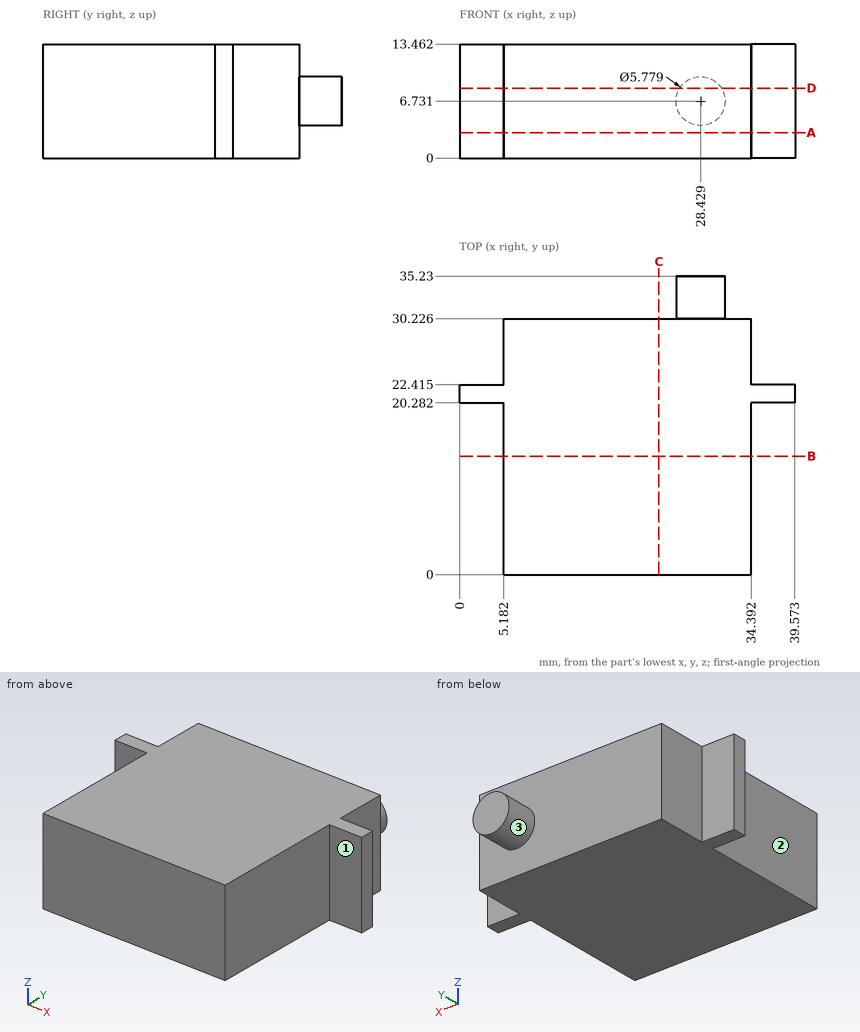
Print and shaded views of the part. All mm, measured from the part's lowest x, y and z. A direction names the side the tool comes from. Round coordinates to 2 decimals unless told otherwise and drop trailing zeros. Write each loop counter-clockwise with the first axis right and the second up, starting at its lowest first coordinate (ties: lowest second). Pieces come first, ordered by that corner, then holes. Notation, with made-up numbers: M 29,46.5 L 78,46.5 A14 ccw 78,59.5 Z; hole C 13,31 d4. An arc over 180 degrees is marked long. Use a Markdown table: item, result. Add a question column.
1. Slice it at D-D on z = 8.25. Give the cut face in (x, y) (1 decimal).
2. Slice it at B-B on y = 14. Give the cut face in (x, z), then the cut area to 3 significant figures.
3. Flat gauge pins, fed straight in: P1, Ø6.5, axis at y = 11.5, z = 7, coming from the +X side; P2, Ø4, axis at x = 2.5, z = 5, coming from the +Y side (1 decimal); P3, Ø5, axis at x = 11, z = 6, coming from the +Y side. Where does each tip first touch, or does it go through?
4. Slice it at C-C on x = 23.5. Give the cut face in (y, z) (1 decimal).
5. Drill centre lines: probe 1 along X at (y, z) = (24, 8.5); probe 2 along Y at (x, z) = (4.5, 11.5) (1 decimal); probe 3 along Y at (x, z) = (18, 4.5) (1 decimal). Where is each one in solid material? Low to high.
6. Slice it at A-A on z = 3. Give the cut face in (x, y) (1 decimal), then the cut area to 3 significant figures.
7. 3-axis set-ups, long thin cutter, end or side, ignore diameter. For the marked faces 1, 2 and 3: which of +Z, -Z, +X, -X, +Y, -Y reach the whole face in a straight line?
Reply:
| question | item | result |
|---|---|---|
| 1 | outline | M 0,20.3 L 5.2,20.3 L 5.2,0 L 34.4,0 L 34.4,20.3 L 39.6,20.3 L 39.6,22.4 L 34.4,22.4 L 34.4,30.2 L 30.9,30.2 L 30.9,35.2 L 26,35.2 L 26,30.2 L 5.2,30.2 L 5.2,22.4 L 0,22.4 Z |
| 2 | outline | M 5.18,0 L 34.39,0 L 34.39,13.46 L 5.18,13.46 Z |
| 2 | area | 393 mm^2 |
| 3 | P1 | stops at x = 34.39 |
| 3 | P2 | stops at y = 22.4 |
| 3 | P3 | stops at y = 30.23 |
| 4 | outline | M 0,0 L 30.2,0 L 30.2,13.5 L 0,13.5 Z |
| 5 | probe 1 | x = 5.18 to 34.39 |
| 5 | probe 2 | y = 20.3 to 22.4 |
| 5 | probe 3 | y = 0 to 30.2 |
| 6 | outline | M 0,20.3 L 5.2,20.3 L 5.2,0 L 34.4,0 L 34.4,20.3 L 39.6,20.3 L 39.6,22.4 L 34.4,22.4 L 34.4,30.2 L 5.2,30.2 L 5.2,22.4 L 0,22.4 Z |
| 6 | area | 905 mm^2 |
| 7 | face 1 | +Z, -Z, +X, -Y |
| 7 | face 2 | +Z, -Z, -X, -Y |
| 7 | face 3 | +Y |
